```python
from build123d import *

# Parameters (mm, degrees)
SKETCH1_R           = 28
SKETCH1_R_2         = 4
SKETCH1_R_3         = 1.5
BOSS_EXTRUDE1_DEPTH = 7
SKETCH2_R           = 25
SKETCH2_R_2         = 18
BOSS_EXTRUDE2_DEPTH = 3
SKETCH3_R           = 1
CUT_EXTRUDE1_DEPTH  = 10


with BuildPart() as part:
    # Sketch1 → Boss-Extrude1 (new body)
    with BuildSketch(Plane.XY):
        Circle(SKETCH1_R)
        Circle(SKETCH1_R_2, mode=Mode.SUBTRACT)
        with Locations((0, 14)):
            Circle(SKETCH1_R_3, mode=Mode.SUBTRACT)
        with Locations((14, 0)):
            Circle(SKETCH1_R_3, mode=Mode.SUBTRACT)
        with Locations((0, -14)):
            Circle(SKETCH1_R_3, mode=Mode.SUBTRACT)
        with Locations((-14, 0)):
            Circle(SKETCH1_R_3, mode=Mode.SUBTRACT)
    extrude(amount=BOSS_EXTRUDE1_DEPTH)

    # Sketch2 → Boss-Extrude2 (add)
    with BuildSketch(Plane(origin=(0, 0, 0), x_dir=(-1, 0, 0), z_dir=(0, 0, -1))):
        with Locations(Location((0, 0, 0), (0, 0, 180))):
            Circle(SKETCH2_R)
        Circle(SKETCH2_R_2, mode=Mode.SUBTRACT)
    extrude(amount=BOSS_EXTRUDE2_DEPTH)

    # Sketch3 → Cut-Extrude1 (cut)
    with BuildSketch(Plane(origin=(0, 0, -3), x_dir=(-1, 0, 0), z_dir=(0, 0, -1))):
        with Locations((-10.75, 18.619546181)):
            Circle(SKETCH3_R)
        with Locations((10.75, 18.619546181)):
            Circle(SKETCH3_R)
        with Locations((21.5, 0)):
            Circle(SKETCH3_R)
        with Locations((10.75, -18.619546181)):
            Circle(SKETCH3_R)
        with Locations((-10.75, -18.619546181)):
            Circle(SKETCH3_R)
        with Locations((-21.5, 0)):
            Circle(SKETCH3_R)
    extrude(amount=-CUT_EXTRUDE1_DEPTH, mode=Mode.SUBTRACT)


solid = part.part
```
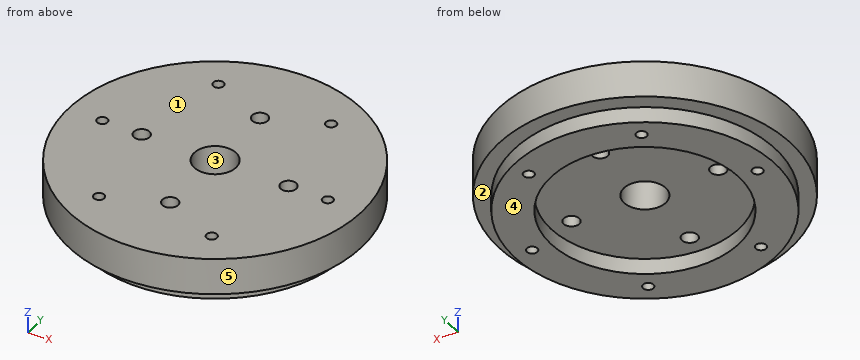
CAD build for the part. Positions are in the model's coordinates, mm. Face numbers are marked on the shaded views. A direction names the side the tool comes from. Round coordinates to 2 decimals unless told otherwise and drop trailing zeros. Order: outer loops, then holes, each group sorted by start corner. A loop starts at its lowest first (then second) coordinate and runs counter-clockwise, first axis right, second up. Notation, with made-up numbers: (19, -5.75) - (49, -5.75) arc R12 cw to (49, 6.25) - close; hole circle Ø6 at (81, -17). An arc over 180 degrees is marked (long way). Answer as CSV lines item,"result". Start each with the question number.
1. Saw through at C-C, the plane z = 2.5. Count the separate pieces of the cut face and the enclosed holes in it, and give its area (3 significant figures).
2. Drill centre lines: L1, parallel to Y at x = 0, z = 2; L2, parallel to Y at x = 11, z = 4.25; L3, parallel to X at y = -3, z = 6.5. Where is each one in solid material? Low to high. Write a range as [from, to].
3. Saw through at D-D, the plane x = -21.5. Write the cut outline in (y, z), and give its area (3 significant figures).
4. Saw through at A-A, the plane x = 0. Write the cut outline in (y, z), and give its area (3 significant figures).
5. Saw through at B-B, the plane y = -14. Write the cut outline in (x, z).
6. Pull direction Y, two halves, no side cores. Call the marked faces 3, 4 and 5: +Y half, -Y half, draft (parallel to the pull), parting line (faces both ways), or undercut.
7. Tool access for the marked faces 1 and 2: list every direction of +Z, -Z, +X, -X, +Y, -Y with a clear straight run to the whole face (end or side of a thin tool).
8. Pin check, flat tips, straight feed: pin 1 (1 mm diameter, centred on x = 9, z = 1.5, fed in from +Y); pin 2 (9 mm diameter, centred on x = 0, y = 0, fed in from -Z); pin 3 (1.5 mm diameter, centred on y = -13, z = -1, fed in from -X). Stop position of each tip, or through.
Model answer:
1,separate pieces,"1"
1,enclosed holes,"11"
1,area,"2,370 mm²"
2,L1,"y = [-28, -15.5], [-12.5, -4], [4, 12.5], [15.5, 28]"
2,L2,"y = [-25.75, -19.59], [-17.65, 17.65], [19.59, 25.75]"
2,L3,"x = [-27.84, -2.65], [2.65, 27.84]"
3,outline,"(-17.94, 0) - (-12.76, 0) - (-12.76, -3) - (-1, -3) - (-1, 7) - (-17.94, 7) - close; (1, -3) - (12.76, -3) - (12.76, 0) - (17.94, 0) - (17.94, 7) - (1, 7) - close"
3,area,"308 mm²"
4,outline,"(-28, 0) - (-25, 0) - (-25, -3) - (-18, -3) - (-18, 0) - (-15.5, 0) - (-15.5, 7) - (-28, 7) - close; (-12.5, 0) - (-4, 0) - (-4, 7) - (-12.5, 7) - close; (4, 0) - (12.5, 0) - (12.5, 7) - (4, 7) - close; (15.5, 0) - (18, 0) - (18, -3) - (25, -3) - (25, 0) - (28, 0) - (28, 7) - (15.5, 7) - close"
4,area,"336 mm²"
5,outline,"(-24.25, 0) - (-20.71, 0) - (-20.71, -3) - (-11.31, -3) - (-11.31, 0) - (-1.5, 0) - (-1.5, 7) - (-24.25, 7) - close; (1.5, 0) - (11.31, 0) - (11.31, -3) - (20.71, -3) - (20.71, 0) - (24.25, 0) - (24.25, 7) - (1.5, 7) - close"
6,face 3,"undercut"
6,face 4,"draft"
6,face 5,"parting line"
7,face 1,"+Z, +X, -X, +Y, -Y"
7,face 2,"-Z"
8,pin 1,"stops at y = 26.68"
8,pin 2,"stops at z = 0"
8,pin 3,"stops at x = -21.79"
